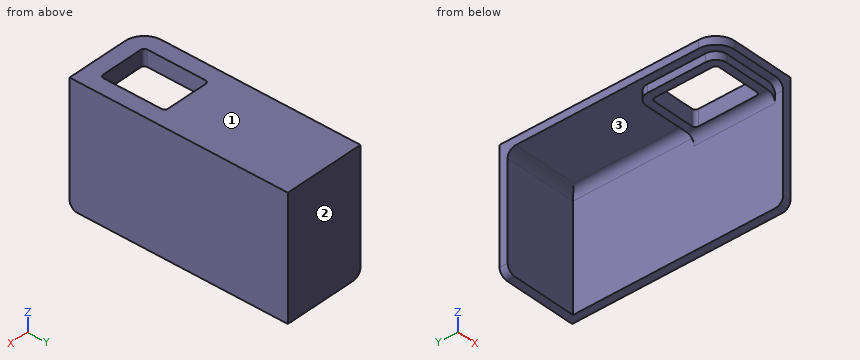
from build123d import *

# Parameters (mm, degrees)
F1_DEPTH = 5
F2_DEPTH = 10
F3_DEPTH = 75
F4_R     = 4.99999


# Not quite as in the source:
# - a fillet or chamfer is up to 0.001 mm smaller than in the source, because OpenCascade refuses the exact size


with BuildPart() as f1:
    # F0 (on Top) → F1 (new body)
    with BuildSketch(Plane.XY):
        with BuildLine():
            ThreePointArc((-20.1, 18.05), (-18.0497474683, 22.9997474683), (-13.1, 25.05))
            Line((-13.1, 25.05), (20.1, 25.05))
            Line((20.1, 25.05), (20.1, 100.05))
            Line((20.1, 100.05), (-25.1, 100.05))
            Line((-25.1, 100.05), (-25.1, -18.05))
            ThreePointArc((-25.1, -18.05), (-21.5852813742, -26.5352813742), (-13.1, -30.05))
            Line((-13.1, -30.05), (20.1, -30.05))
            Line((20.1, -30.05), (20.1, -25.05))
            Line((20.1, -25.05), (-13.1, -25.05))
            ThreePointArc((-13.1, -25.05), (-18.0497474683, -22.9997474683), (-20.1, -18.05))
            Line((-20.1, -18.05), (-20.1, 18.05))
        make_face()
    extrude(amount=-F1_DEPTH)

    # F0 (on Top) → F2 (join)
    with BuildSketch(Plane.XY):
        with BuildLine():
            Line((20.1, 25.05), (-13.1, 25.05))
            ThreePointArc((-13.1, 25.05), (-18.0497474683, 22.9997474683), (-20.1, 18.05))
            Line((-20.1, 18.05), (-20.1, -18.05))
            ThreePointArc((-20.1, -18.05), (-18.0497474683, -22.9997474683), (-13.1, -25.05))
            Line((-13.1, -25.05), (20.1, -25.05))
            Line((20.1, -25.05), (20.1, 25.05))
        make_face()
        with BuildLine():
            Line((-13.1, 20.05), (13.1, 20.05))
            ThreePointArc((13.1, 20.05), (14.5142135624, 19.4642135624), (15.1, 18.05))
            Line((15.1, 18.05), (15.1, -18.05))
            ThreePointArc((15.1, -18.05), (14.5142135624, -19.4642135624), (13.1, -20.05))
            Line((13.1, -20.05), (-13.1, -20.05))
            ThreePointArc((-13.1, -20.05), (-14.5142135624, -19.4642135624), (-15.1, -18.05))
            Line((-15.1, -18.05), (-15.1, 18.05))
            ThreePointArc((-15.1, 18.05), (-14.5142135624, 19.4642135624), (-13.1, 20.05))
        make_face(mode=Mode.SUBTRACT)
    extrude(amount=-F2_DEPTH)

    # F0 (on Top) → F3 (join)
    with BuildSketch(Plane.XY):
        Polygon((20.1, 100.05), (20.1, 25.05), (20.1, -25.05), (20.1, -30.05), (25.1, -30.05), (25.1, 105.05), (-25.1, 105.05), (-25.1, 100.05), align=None)
    extrude(amount=-F3_DEPTH)

    # F4 (radius 5 in the source; OpenCascade refuses exactly that, so slightly less here)
    f4_edges = [f1.edges().sort_by_distance(p)[0] for p in [
        (20.1, -27.55, -5),
        (20.1, 62.55, -5),
        (20.1, 0, -10),
        (22.6, -30.05, -75),
        (-25.1, 102.55, -75),
        (-2.5, 100.05, -5),
    ]]
    fillet(f4_edges, radius=F4_R)


solid = f1.part
Check sheet for the modelled part. Datum: model origin and axes. Units: mm. Face numbers are marked on the shaded views. Round coordinates to 2 decimals unless told otherwise and drop trailing zeros. Loops run counter-clockwise (first coordinate to the right, second up) from the corner with the lowest first, then second, coordinate; pieces in that order, holes last. Notation, with made-up numbers: (46.5, 66.5) - (93.5, 66.5) arc R13 cw to (93.5, 83.5) - close; hole circle Ø3 at (21, -37). An arc over 180 degrees is marked (long way). Answer as CSV lines item,"result". Start each with the question number.
Item 1: Release check for a two-part mould opening along Y. For the marked faces 1, 2 and 3 record: +Y half, -Y half, draft (parallel to the pull), parting line (faces both ways), or undercut.
Item 2: Depth check by flat-ended pin: P1, Ø11, axis at x = 10, z = -11.5, coming from the -Y side; P2, Ø12, axis at y = 41.5, z = -27, coming from the -X side; P3, Ø2, axis at x = -2, z = -52.5, coming from the -Y side; P4, Ø10.5, axis at x = -2, y = -10, coming from the -Z side. Enter the tip coordinate at first touch or a pass-through.
Item 3: Section check C-C (z = -7). Record the boundary of the cut face in (x, y), and give its area (3 significant figures).
Item 4: Section check B-B (x = -2.5). Record the boundary of the cut face in (y, z), and give its area (3 significant figures).
Item 5: Scan lines: line 1 (X direction, y = 65.5, z = -25.5); line 2 (Y direction, x = 10, z = -58); line 3 (Z direction, x = -5, y = 87.5). Record each from-to range of solid material in increasing order. Write a range as [from, to].
Item 6: Section check D-D (y = 31). Record the boundary of the cut face in (x, z), and give its area (3 significant figures).
Report:
1,face 1,"draft"
1,face 2,"+Y half"
1,face 3,"undercut"
2,P1,"stops at y = -25.05"
2,P2,"stops at x = 20.1"
2,P3,"stops at y = 100.05"
2,P4,"passes through"
3,outline,"(-25.1, 99.05) - (19.1, 99.05) - (19.1, 25.05) - (-13.1, 25.05) arc R7 ccw to (-20.1, 18.05) - (-20.1, -18.05) arc R7 ccw to (-13.1, -25.05) - (19.1, -25.05) - (19.1, -30.05) - (25.1, -30.05) - (25.1, 105.05) - (-25.1, 105.05) - close; hole (-15.1, -18.05) arc R2 ccw to (-13.1, -20.05) - (13.1, -20.05) arc R2 ccw to (15.1, -18.05) - (15.1, 18.05) arc R2 ccw to (13.1, 20.05) - (-13.1, 20.05) arc R2 ccw to (-15.1, 18.05) - close"
3,area,"1,810 mm2"
4,outline,"(-30.05, -5) - (-25.05, -5) - (-25.05, -10) - (-20.05, -10) - (-20.05, 0) - (-30.05, 0) - close; (20.05, -10) - (25.05, -10) - (25.05, -5) - (95.05, -5) arc R5 cw to (100.05, -10) - (100.05, -75) - (105.05, -75) - (105.05, 0) - (20.05, 0) - close"
4,area,"880 mm2"
5,line 1,"x = [20.1, 25.1]"
5,line 2,"y = [100.05, 105.05]"
5,line 3,"z = [-5, 0]"
6,outline,"(-25.1, -5) - (15.1, -5) arc R5 cw to (20.1, -10) - (20.1, -75) - (25.1, -75) - (25.1, 0) - (-25.1, 0) - close"
6,area,"606 mm2"
